CAD build for the part. Positions are in the model's coordinates, mm. A direction names the side the tool comes from. Coordinates: 2 decimals unless noted, no trailing zeros. Order: outer loops, then holes, each group sorted by start corner. A loop starts at its lowest first (then second) coordinate and runs counter-clockwise, first axis right, second up. Notation, with made-up numbers: (24, -29.5) - (31, -29.5) arc R28 cw to (31, 1.5) - close; hole circle Ø7 at (73, 33). An arc over 180 degrees is marked (long way). Write each question's results on one line, items separated by ' | '. Start each with the question number.
Q1. Pin check, flat tips, straight feed: P1, Ø0.9, axis at x = -247, z = -5, coming from the -Y side; P2, Ø1.5, axis at y = 8, z = -4, coming from the -X side; P3, Ø8, axis at x = -99, y = 43.5, coming from the +Z side; P4, Ø0.9, axis at y = -6, z = -4.5, coming from the -X side. Stop position of each tip, or through.
Q2. Pull direction X, two halves, no side cores. Call faces 3 (the flat face through (-69, 21, -3)), 4 (the flat face through (54.69, 23.95, -4.48)): released by +X, released by -X, zero draft, split by the parting line, or undercut.
Q3. Wall check: probe 1 along X at (y, z) = (32.5, -4.05); probe 2 along Y at (x, z) = (-189, -4.5); probe 3 along Y at (x, z) = (-137, -4.1). Give the ranges that are in metal, low to high.
Q4. Which spindle directions (+Z, -Z, +X, -X, +Y, -Y) get a long thin tool onto all of the face, cutting with end or side? Do faces 1 (the flat face through (-69, 21, -6)), 2 (the flat face through (-195.93, 12.636, -4.479)). Say none if no direction does.
Q5. Band-saw the part on A-A, the plane y = 38. Write the cut outline in (x, z), then the cut area to 3 significant figures.
Q6. Band-saw the part on C-C, the plane z = -3.6. Count the separate pieces of the cut face and the enclosed holes in it, then the cut area to 3 significant figures.
Q7. Band-saw the part on B-B, the plane x = 71. Write the cut outline in (y, z).
```python
from build123d import *

# Parameters (mm, degrees)
BOSS_EXTRUDE2_DEPTH = 3


with BuildPart() as part:
    # Sketch6 → Boss-Extrude2 (new body)
    with BuildSketch(Plane(origin=(0, 0, -3), x_dir=(-1, 0, 0), z_dir=(0, 0, -1))):
        with BuildLine():
            Line((-19.25, 3.741713812), (0, -0.35))
            add(Edge.make_bspline(
                [(0, -0.35), (3.178862469, 6.495343287), (8.987756305, 8.032168144), (22.140633739, 13.071207305), (43.250433247, 17.69324185), (66.39602757, 18.219905629)],
                knots=[0, 0, 0, 0, 0, 0, 1, 1, 1, 1, 1, 1], degree=5))
            add(Edge.make_bspline(
                [(66.39602757, 18.219905629), (73.079858249, 18.217137873), (79.768873399, 18.101745103), (86.45, 17.815976098)],
                knots=[0.875945967, 0.875945967, 0.875945967, 0.875945967, 0.985673704, 0.985673704, 0.985673704, 0.985673704], degree=3))
            Line((86.45, 17.815976098), (86.45, 24.670250599))
            Line((86.45, 24.670250599), (89.45, 24.670250599))
            Line((89.45, 24.670250599), (89.45, 17.675984992))
            add(Edge.make_bspline(
                [(89.45, 17.675984992), (90.320899947, 17.631898595), (91.191632468, 17.584767892), (92.062168571, 17.534464817)],
                knots=[1.002100386, 1.002100386, 1.002100386, 1.002100386, 1.01640933, 1.01640933, 1.01640933, 1.01640933], degree=3))
            add(Edge.make_bspline(
                [(92.062168571, 17.534464817), (95.665977641, 17.334138157), (108.464938821, 16.428798519), (140.620964858, 12.117510077), (188.052718325, 1.033122833), (227.303556849, -4.3666315), (246.35, -10.231818509)],
                knots=[0, 0, 0, 0, 0.05922822, 0.210539222, 0.531730365, 0.858409316, 0.858409316, 0.858409316, 0.858409316], degree=3))
            Line((246.35, -10.231818509), (246.35, -4.231818509))
            Line((246.35, -4.231818509), (249.35, -4.231818509))
            Line((249.35, -4.231818509), (249.35, -10.422260297))
            Line((249.35, -10.422260297), (261.434958207, -8.613902826))
            Line((261.434958207, -8.613902826), (261.434958207, -0.35))
            Line((261.434958207, -0.35), (254.27, -1.277143049))
            Line((254.27, -1.277143049), (254.27, 49.289954404))
            Line((254.27, 49.289954404), (264.27, 48.703684462))
            Line((264.27, 48.703684462), (264.27, 57.518794836))
            Line((264.27, 57.518794836), (254.27, 58.105064779))
            Line((254.27, 58.105064779), (249.35, 58.39350959))
            Line((249.35, 58.39350959), (249.35, 52.569390573))
            Line((249.35, 52.569390573), (246.35, 52.569390573))
            Line((246.35, 52.569390573), (246.35, 58.569390573))
            Line((246.35, 58.569390573), (174.35, 62.790534157))
            Line((174.35, 62.790534157), (174.35, 57.781948717))
            Line((174.35, 57.781948717), (159.35, 58.66135363))
            Line((159.35, 58.66135363), (159.35, 63.66993907))
            Line((159.35, 63.66993907), (118.45, 66.067783134))
            Line((118.45, 66.067783134), (118.45, 61.560056238))
            Line((118.45, 61.560056238), (104.45, 62.380834157))
            Line((104.45, 62.380834157), (104.45, 66.888561053))
            Line((104.45, 66.888561053), (89.45, 67.767965967))
            Line((89.45, 67.767965967), (89.45, 62.370250599))
            Line((89.45, 62.370250599), (86.45, 62.370250599))
            Line((86.45, 62.370250599), (86.45, 68.043292799))
            Line((86.45, 68.043292799), (-16.333378442, 66.994986377))
            Line((-16.333378442, 66.994986377), (-19.25, 66.904044127))
            Line((-19.25, 66.904044127), (-19.25, 60.904044127))
            Line((-19.25, 60.904044127), (-22.25, 60.904044127))
            Line((-22.25, 60.904044127), (-22.25, 66.810502081))
            Line((-22.25, 66.810502081), (-111.531056313, 64.026657849))
            Line((-111.531056313, 64.026657849), (-121.52619868, 63.715002493))
            Line((-121.52619868, 63.715002493), (-121.52619868, 25.481190944))
            Line((-121.52619868, 25.481190944), (-111.531056313, 23.356657849))
            Line((-111.531056313, 23.356657849), (-22.25, 4.379383497))
            Line((-22.25, 4.379383497), (-22.25, 9.741713812))
            Line((-22.25, 9.741713812), (-19.25, 9.741713812))
            Line((-19.25, 9.741713812), (-19.25, 3.741713812))
        make_face()
        Polygon((-84.1, 54.203030213), (-26.1, 57.75847956), (-26.1, 17.874749636), (-84.1, 30.203030213), align=None, mode=Mode.SUBTRACT)
        with BuildLine():
            Line((-10.5, 21.65), (-10.5, 55.95))
            Line((-10.5, 55.95), (87.47, 56.949213898))
            Line((87.47, 56.949213898), (87.47, 30.129694509))
            ThreePointArc((87.47, 30.129694509), (86.67270256, 28.299174366), (84.789356805, 27.636229443))
            add(Edge.make_bspline(
                [(14.701665666, 21.959575817), (21.19900444, 24.808951329), (34.471850374, 27.925627057), (54.295468051, 29.219545771), (70.832055402, 28.62299092), (81.026620283, 27.908827105), (84.789356805, 27.636229443)],
                knots=[0.099500985, 0.099500985, 0.099500985, 0.099500985, 0.360279093, 0.592189537, 0.828480504, 0.96707438, 0.96707438, 0.96707438, 0.96707438], degree=3))
            Line((14.701665666, 21.959575817), (7.522354632, 18.142268428))
            Line((7.522354632, 18.142268428), (0, 21.65))
            Line((0, 21.65), (0, 16.35))
            Line((0, 16.35), (-3, 16.35))
            Line((-3, 16.35), (-3, 21.65))
            Line((-3, 21.65), (-10.5, 21.65))
        make_face(mode=Mode.SUBTRACT)
        Polygon((93.97, 30.170250599), (93.97, 55.670250599), (238.97, 45.483901662), (238.97, 9.104044127), (220.823057098, 7.643571), (170.32923345, 17.7710139), align=None, mode=Mode.SUBTRACT)
    extrude(amount=BOSS_EXTRUDE2_DEPTH)


solid = part.part
```
Results below:
1) P1: stops at y = -4.23 | P2: stops at x = -254.27 | P3: passes through | P4: stops at x = -261.43
2) face 3: zero draft | face 4: undercut
3) probe 1: x = -254.27 to -238.97, -93.97 to -87.47, 10.5 to 26.1, 84.1 to 121.53 | probe 2: y = 1.79 to 14.03, 48.99 to 61.93 | probe 3: y = 12.06 to 23.18, 52.65 to 64.98
4) face 1: -Z, +X, -X, +Y, -Y | face 2: +Z, -Z
5) outline: (-254.27, -6) - (-238.97, -6) - (-238.97, -3) - (-254.27, -3) - close; (-93.97, -6) - (-87.47, -6) - (-87.47, -3) - (-93.97, -3) - close; (10.5, -6) - (26.1, -6) - (26.1, -3) - (10.5, -3) - close; (84.1, -6) - (121.53, -6) - (121.53, -3) - (84.1, -3) - close | area: 224 mm²
6) separate pieces: 1 | enclosed holes: 3 | area: 11,100 mm²
7) outline: (14.74, -6) - (27.42, -6) - (27.42, -3) - (14.74, -3) - close; (55.01, -6) - (65.29, -6) - (65.29, -3) - (55.01, -3) - close
